Source: CAD feature listing. Evaluate the final solid. Frame: model axes, mm. Face numbers are marked on the shaded views. A direction names the side the tool comes from. Give positions to 0.01 mm unless a question says otherwise; leave off trailing zeros. Order: outer loops, then holes, each group sorted by start corner. A loop starts at its lowest first (then second) coordinate and runs counter-clockwise, first axis right, second up. Notation, with made-up numbers: (81, 71.25) -> (122, 71.25) arc R24 cw to (122, 104.25) -> close; hole circle Ø10 at (-39.5, 18). An arc over 180 degrees is marked (long way). Answer in a Markdown table with one row per item.
Autodesk Inventor part; units mm, degrees
ref_plane "YZ Plane" through (0, 0, 0) normal (1, 0, 0) x (0, 1, 0)
ref_plane "XZ Plane" through (0, 0, 0) normal (0, 1, 0) x (-1, 0, 0)
ref_plane "XY Plane" through (0, 0, 0) normal (0, 0, 1) x (1, 0, 0)
sketch "Sketch1" plane through (0, 0, 0) normal (0, 1, 0) x (-1, 0, 0)
  line L0 (-110, 55) -> (110, 55)
  line L1 (110, 55) -> (110, -55)
  line L2 (110, -55) -> (-110, -55)
  line L3 (-110, -55) -> (-110, 55)
  line L4 (-110, 55) -> (110, -55) construction
  line L5 (110, 55) -> (-110, -55) construction
  line L6 (-150, 100) -> (150, 100)
  line L7 (150, 100) -> (150, -100)
  line L8 (150, -100) -> (-150, -100)
  line L9 (-150, -100) -> (-150, 100)
  line L10 (-150, 100) -> (150, -100) construction
  line L11 (150, 100) -> (-150, -100) construction
  point P0 (0, 0)
  dimension "d0" = 220
  dimension "d1" = 110
  dimension "d2" = 300
  dimension "d3" = 200
extrude "Extrusion1" add sketch "Sketch1" along normal blind 10 contours L0 L1 L2 L3
extrude "Extrusion2" add sketch "Sketch1" along normal blind 40
sketch "Sketch2" plane through (-150, 0, 100) normal (0, 0, 1) x (1, 0, 0)
  line L0 (300, 0) -> (0, 0)
  line L1 (300, 0) -> (300, 40)
  line L2 (0, 0) -> (300, 0)
  line L3 (300, 0) -> (300, 40)
  line L4 (300, 40) -> (0, 40)
  line L5 (0, 40) -> (0, 0)
  circle A0 centre (70, 20) radius 50
  point P0 (150, 0)
  dimension "d8" = 100
sketch "Sketch3" plane through (150, 0, -100) normal (0, 0, -1) x (-1, 0, 0)
  line L0 (300, 0) -> (300, 40)
  line L1 (0, 40) -> (300, 40)
  line L2 (300, 0) -> (0, 0)
  line L3 (0, 0) -> (0, 40)
  line L4 (0, 40) -> (300, 40)
  line L5 (300, 40) -> (300, 0)
  line L6 (300, 0) -> (230, 0) construction
  line L7 (230, 0) -> (230, 20) construction
  line L8 (230, 20) -> (300, 20) construction
  line L9 (300, 20) -> (300, 0) construction
  circle A0 centre (230, 20) radius 50
  point P0 (150, 0)
  dimension "d9" = 70
  dimension "d10" = 20
  dimension "d11" = 100
extrude "Extrusion3" add sketch "Sketch3" along normal blind 25 contours A0 L2 | L2 A0 L1 | L1 A0
extrude "Extrusion4" add sketch "Sketch2" along normal blind 25 contours A0 L0 | L0 A0 L4 | L4 A0
properties part number "Chassis"
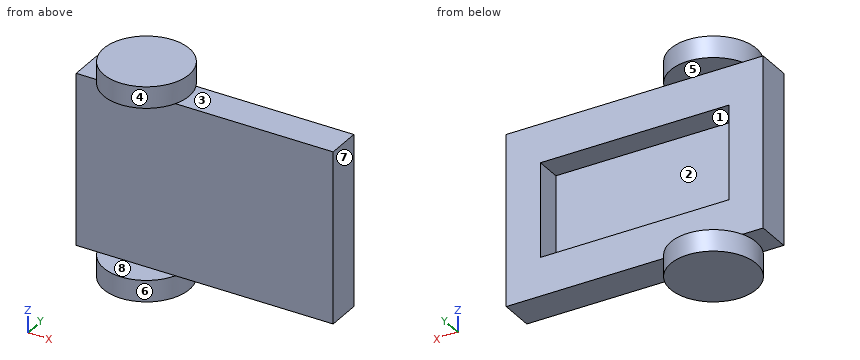
(1) Section query C-C (y = 20). Return the cut outline in (x, z).
A:
| item | result |
|---|---|
| outline | (-150, -100) -> (-130, -100) -> (-130, -125) -> (-30, -125) -> (-30, -100) -> (150, -100) -> (150, 100) -> (-30, 100) -> (-30, 125) -> (-130, 125) -> (-130, 100) -> (-150, 100) -> close; hole (-110, -55) -> (110, -55) -> (110, 55) -> (-110, 55) -> close |
(2) First-contact query: pin 1 Ø7.5 at (x, y) = (-136, 24.5) entering from -Z; pin 2 Ø9 at (x, y) = (-24, 30.5) entering from +Z; pin 3 Ø6 at (x, z) = (80.5, 65) entering from -Y; pin 4 Ø12 at (x, y) = (-133, 10) entering from +Z. Flat tips, straight axial feed; report the tip coordinate or a pass-through.
A:
| item | result |
|---|---|
| pin 1 | stops at z = -100 |
| pin 2 | stops at z = 100 |
| pin 3 | stops at y = 0 |
| pin 4 | stops at z = 125 |
(3) Ray query, probe 1 along Z at (x, y) = (104.5, 38.5); probe 2 along Z at (x, y) = (-52, -5); probe 3 along X at (y, z) = (12.5, -7.5). Return the intervals inside material, ascending.
A:
| item | result |
|---|---|
| probe 1 | z = -100 to -55, 55 to 100 |
| probe 2 | z = -125 to -100, 100 to 125 |
| probe 3 | x = -150 to -110, 110 to 150 |
(4) Access query for the marked faces 5, 6, 7 and 8. Directions: +Z, -Z, +X, -X, +Y, -Y. A direction counts if a zero-diameter tool reaches every point of the face in a straight line with its end or side. Return the directions, or none.
A:
| item | result |
|---|---|
| face 5 | +X, -X, +Y |
| face 6 | -Z |
| face 7 | +Z, -Z, +X, +Y, -Y |
| face 8 | +X, -X, -Y |
(5) Section query A-A (y = -10). Return the cut outline in (x, z), plus the area to 3 significant figures.
A:
| item | result |
|---|---|
| outline | (-120, -125) -> (-40, -125) -> (-40, -100) -> (-120, -100) -> close; (-120, 100) -> (-40, 100) -> (-40, 125) -> (-120, 125) -> close |
| area | 4,000 mm^2 |
(6) Pull-direction query (X, two-part tool) for the marked faces 1, 2, 3 and 4; classes: +X half, -X half, draft (parallel to the pull), parting line (faces both ways), or undercut.
A:
| item | result |
|---|---|
| face 1 | undercut |
| face 2 | undercut |
| face 3 | draft |
| face 4 | parting line |
(7) Section query D-D (z = 45.5). Return the cut outline in (x, y), plus the area to 3 significant figures.
A:
| item | result |
|---|---|
| outline | (-150, 0) -> (150, 0) -> (150, 40) -> (110, 40) -> (110, 10) -> (-110, 10) -> (-110, 40) -> (-150, 40) -> close |
| area | 5,400 mm^2 |
(8) Section query B-B (x = -80). Return the cut outline in (y, z), plus the area to 3 significant figures.
A:
| item | result |
|---|---|
| outline | (-30, -125) -> (70, -125) -> (70, -100) -> (40, -100) -> (40, -55) -> (10, -55) -> (10, 55) -> (40, 55) -> (40, 100) -> (70, 100) -> (70, 125) -> (-30, 125) -> (-30, 100) -> (0, 100) -> (0, -100) -> (-30, -100) -> close |
| area | 9,700 mm^2 |
